```python
from build123d import *

# Parameters (mm, degrees)
PAD_DEPTH         = 1
PAD001_DEPTH      = 6.8
PAD001_DEPTH_BACK = 6.8
CYLINDER_R        = 0.4
CYLINDER_DEPTH    = 13.6
CYLINDER003_R     = 2.5
CYLINDER003_DEPTH = 0.6
CYLINDER004_R     = 0.8
CYLINDER004_DEPTH = 0.4
CHAMFER_SIZE      = 0.4


with BuildPart() as part:
    # Sketch → Pad (new body)
    with BuildSketch(Plane.XY):
        with BuildLine():
            Line((0, 10), (80, 10))
            Line((80, 10), (80, -10))
            Line((0, -10), (80, -10))
            ThreePointArc((0, 10), (-10, 0), (0, -10))
        make_face()
    extrude(amount=PAD_DEPTH)

    # Sketch003 (on Sketch) → Pad001 (join, two sides)
    with BuildSketch(Plane.XZ) as pad001_sk:
        with BuildLine():
            Line((80, 0), (82.25, 0))
            ThreePointArc((82.25, 0), (83.090481, 2.14888), (80.972274, 1.233843))
            ThreePointArc((80, 1), (80.503859, 1.043236), (80.972274, 1.233843))
            Line((80, 1), (80, 0))
        make_face()
    extrude(amount=PAD001_DEPTH)
    extrude(pad001_sk.sketch, amount=-PAD001_DEPTH_BACK)

    # Cylinder → Cylinder (cut)
    with BuildSketch(Plane(origin=(82.25, 6.8, 1.25), x_dir=(1, 0, 0), z_dir=(0, -1, 0))):
        Circle(CYLINDER_R)
    extrude(amount=CYLINDER_DEPTH, mode=Mode.SUBTRACT)

    # Cylinder003 → Cylinder003 (cut)
    with BuildSketch(Plane.XY):
        Circle(CYLINDER003_R)
    extrude(amount=CYLINDER003_DEPTH, mode=Mode.SUBTRACT)

    # Cylinder004 → Cylinder004 (cut)
    with BuildSketch(Plane.XY.offset(0.6)):
        Circle(CYLINDER004_R)
    extrude(amount=CYLINDER004_DEPTH, mode=Mode.SUBTRACT)

    # Chamfer
    chamfer_edges = [part.edges().sort_by_distance(p)[0] for p in [
        (40, -10, 1),
        (-10, 0, 1),
        (40, 10, 1),
        (40, 10, 0),
        (-10, 0, 0),
        (40, -10, 0),
    ]]
    chamfer(chamfer_edges, length=CHAMFER_SIZE)


solid = part.part
```
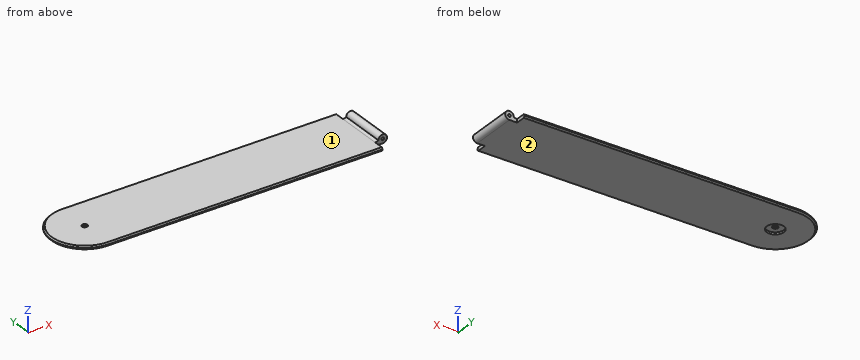
The listing builds one solid part. Answer for the finished solid, in the listing's coordinates (mm). Face numbers are marked on the shaded views. A direction names the side the tool comes from. Round coordinates to 2 decimals unless told otherwise and drop trailing zeros. Loops run counter-clockwise (first coordinate to the right, second up) from the corner with the lowest first, then second, coordinate; pieces in that order, holes last. Notation, with made-up numbers: (-29.5, 52) -> (19.5, 52) arc R11 ccw to (19.5, 58) -> close; hole circle Ø11 at (32, 10.5). An arc over 180 degrees is marked (long way). Use one line per item in the form item = value.
1. The part is cut by section B-B on x = 14.5. Determine the outline of the cut face in (y, z).
Answer key:
outline = (-10, 0.4) -> (-9.6, 0) -> (9.6, 0) -> (10, 0.4) -> (10, 0.6) -> (9.6, 1) -> (-9.6, 1) -> (-10, 0.6) -> close
2. The part is cut by section A-A on y = 0. Determine the outline of the cut face in (x, z), and give its area (3 significant figures).
Answer key:
outline = (-10, 0.4) -> (-9.6, 0) -> (-2.5, 0) -> (-2.5, 0.6) -> (-0.8, 0.6) -> (-0.8, 1) -> (-9.6, 1) -> (-10, 0.6) -> close; (0.8, 0.6) -> (2.5, 0.6) -> (2.5, 0) -> (82.25, 0) arc R1.25 ccw (long way) to (80.97, 1.23) arc R1.69 cw to (80, 1) -> (0.8, 1) -> close; hole circle Ø0.8 at (82.25, 1.25)
area = 92.0 mm²
3. Flat-ended cylindrical pins translate along their axes: pin 1 Ø1.1 at (y, z) = (-9, 0.5) entering from +X; pin 2 Ø1.4 at (x, y) = (0, 0) entering from -Z; pin 3 Ø8 at (x, y) = (0, 0) entering from -Z; pin 4 Ø3 at (x, y) = (9, -7) entering from +Z. Find the tip coordinate at first contact, or state that the pin passes through.
Answer key:
pin_1 = 80
pin_2 = through
pin_3 = 0
pin_4 = 1
4. The part is cut by section C-C on z = 2.1. Determine the outline of the cut face in (x, y), and give its area (3 significant figures).
Answer key:
outline = (81.31, -6.8) -> (83.14, -6.8) -> (83.14, 6.8) -> (81.31, 6.8) -> close
area = 24.9 mm²
5. A tool of negligible diameter and unlimited length cuts with its end or side. For the marked faces 1 and 2, from which of +Z, -Z, +X, -X, +Y, -Y can it reach the whole face along a straight path? Write none if from no direction.
Answer key:
face_1 = +Z, -X, +Y, -Y
face_2 = -Z, +X, -X, +Y, -Y
6. Find the intervals of material crossed by probe 1 along Z at (x, y) = (82.25, -2.5); probe 2 along Y at (x, z) = (0, 0.4); probe 3 along X at (y, z) = (-1, 1.3), in increasing order. Write a range as [from, to].
Answer key:
probe_1 = [0, 0.85], [1.65, 2.5]
probe_2 = [-10, -2.5], [2.5, 10]
probe_3 = [80.97, 81.85], [82.65, 83.47]
